Could you check a few things on this model? Use its own coordinates, in mm. A direction names the side the tool comes from. Coordinates: 2 decimals unless noted, no trailing zeros. Loops run counter-clockwise (first coordinate to the right, second up) from the corner with the lowest first, then second, coordinate; pieces in that order, holes last.
1) If I drill on line 1 along Y through (x, z) = (0, 2.1); line 2 along Z through (x, y) = (1.85, -0.1); line 3 along X through (y, z) = (-1, 1.5), over which ranges is the centre line in solid material (lowest first)?
2) For faces 4 (the face through (-1.5, 0.07, 2.93)), 5 (the face through (-1.975, -1.119, 2.465)), 6 (the face through (1.5, 0.07, -2.91)), which set-ups out of +Z, -Z, +X, -X, +Y, -Y let a thin tool reach every point of the face, with its end or its side?
3) Imagine slicing it at B-B on z = -3.5. Please give me the cut outline in (x, y), plus the area to 3 significant figures.
4) Thinking about a two-plate mould opening in Y: for faces 1 (the face through (1.957, -1.151, 2.465)), 2 (the face through (0, 0, 1)), 3 (the face through (-1.957, 1.151, 2.465)), which applies, released by +Y, released by -Y, zero draft, split by the parting line, or undercut?
5) Will these pins go through, and if not, where does the flat tip stop? P1, Ø2, axis at y = 0, z = -3, coming from the -X side; P2, Ø0.9, axis at x = 0.5, y = 0, coming from the +Z side; P3, Ø2, axis at y = -1, z = -3.5, coming from the +X side.
6) Imagine slicing it at A-A on z = 4. Please give me the cut outline in (x, y).
```python
from build123d import *

# Parameters (mm, degrees)
BOSS_EXTRUDE1_DEPTH     = 5
SKETCH2_R               = 1.5
CUT_EXTRUDE1_DEPTH      = 1
CUT_EXTRUDE1_DEPTH_BACK = 4
CHAMFER1_SIZE           = 0.2
SKETCH4_R               = 1.5
BOSS_EXTRUDE2_DEPTH     = 6.5
CHAMFER2_SIZE           = 0.6


with BuildPart() as part:
    # Sketch1 → Boss-Extrude1 (new body)
    with BuildSketch(Plane.XY):
        Polygon((2.621170222, 0), (1.310585111, 2.27), (-1.310585111, 2.27), (-2.621170222, 0), (-1.310585111, -2.27), (1.310585111, -2.27), align=None)
    extrude(amount=BOSS_EXTRUDE1_DEPTH)

    # Sketch2 → Cut-Extrude1 (cut, two sides)
    with BuildSketch(Plane.XY.offset(5)) as cut_extrude1_sk:
        Circle(SKETCH2_R)
    extrude(amount=CUT_EXTRUDE1_DEPTH, mode=Mode.SUBTRACT)
    extrude(cut_extrude1_sk.sketch, amount=-CUT_EXTRUDE1_DEPTH_BACK, mode=Mode.SUBTRACT)

    # Sketch3 → Cut-Revolve1 (revolve, cut)
    with BuildSketch(Plane(origin=(0, 0, 0), x_dir=(1, 0, 0), z_dir=(0, 1, 0))):
        Polygon((-2.621170222, -5), (-2.271170222, -5), (-2.621170222, -4.8), align=None)
    revolve(axis=Axis((0, 0, 1), (0, 0, 1)), mode=Mode.SUBTRACT)

    # Chamfer1
    chamfer1_edges = [part.edges().sort_by_distance(p)[0] for p in [
        (-1.5, 0, 5),
    ]]
    chamfer(chamfer1_edges, length=CHAMFER1_SIZE)

    # Sketch4 → Boss-Extrude2 (add)
    with BuildSketch(Plane(origin=(0, 0, 0), x_dir=(-1, 0, 0), z_dir=(0, 0, -1))):
        Circle(SKETCH4_R)
    extrude(amount=BOSS_EXTRUDE2_DEPTH)

    # Chamfer2
    chamfer2_edges = [part.edges().sort_by_distance(p)[0] for p in [
        (1.5, 0, -6.5),
    ]]
    chamfer(chamfer2_edges, length=CHAMFER2_SIZE)


solid = part.part
```
Filled in:
1. line 1: y = -2.27 to -1.5, 1.5 to 2.27
1. line 2: z = 0 to 5
1. line 3: x = -2.04 to -1.12, 1.12 to 2.04
2. face 4: +Z
2. face 5: +Z, -Z, -X, -Y
2. face 6: -Z
3. outline: circle Ø3 at (0, 0)
3. area: 7.07 mm2
4. face 1: released by -Y
4. face 2: undercut
4. face 3: released by +Y
5. P1: stops at x = -1.5
5. P2: stops at z = 1
5. P3: stops at x = 1.5
6. outline: (-2.62, 0) - (-1.31, -2.27) - (1.31, -2.27) - (2.62, 0) - (1.31, 2.27) - (-1.31, 2.27) - close; hole circle Ø3 at (0, 0)
